For this review, take the finished solid that the model builds, in its own axes (mm). A direction names the side the tool comes from. Coordinates: 2 decimals unless noted, no trailing zeros. Loops run counter-clockwise (first coordinate to the right, second up) from the corner with the lowest first, then second, coordinate; pieces in that order, holes last. Notation, with made-up numbers: M 34,-6.5 L 89,-6.5 A13 cw 89,13.5 Z; hole C 18,79 d10. An arc over 180 degrees is marked long. Write item = value, one per line.
from build123d import *

# Parameters (mm, degrees)
F0_W     = 285
F0_H     = 185
F0_R     = 17.5
F1_DEPTH = 25
F2_SIZE  = 15
F3_T     = -1.5


with BuildPart() as f1:
    # F0 (on Top) → F1 (new body)
    with BuildSketch(Plane.XY):
        with Locations((-142.5, 92.5)):
            Rectangle(F0_W, F0_H)
        with Locations((-142.5, 92.5)):
            Circle(F0_R, mode=Mode.SUBTRACT)
    extrude(amount=F1_DEPTH)

    # F2
    f2_edges = [f1.edges().sort_by_distance(p)[0] for p in [
        (0, 92.5, 25),
        (-142.5, 185, 25),
        (-285, 92.5, 25),
        (-142.5, 0, 25),
    ]]
    chamfer(f2_edges, length=F2_SIZE)

    # F3
    f3_openings = [f1.faces().sort_by_distance(p)[0] for p in [
        (-142.5, 3.397793, 0),
        (-160, 92.5, 12.5),
    ]]
    offset(amount=F3_T, openings=f3_openings)


solid = f1.part
Q1. Draft analysis for pull direction X (two halves, no side actions). For faces 3 (the face through (-144, 185, 5)), 4 (the face through (-277, 91, 18)), 5 (the face through (-144.47, 8.66, 16.54)), 6 (the face through (-8.66, 91.23, 16.54)), state which applies: +X half, -X half, draft (parallel to the pull), parting line (faces both ways), or undercut.
Solved:
face_3 = draft
face_4 = -X half
face_5 = undercut
face_6 = undercut
Q2. Add section D-D (y = 138). Write out the cut boundary in (x, z).
Solved:
outline = M -285,0 L -283.5,0 L -283.5,9.38 L -269.38,23.5 L -15.62,23.5 L -1.5,9.38 L -1.5,0 L 0,0 L 0,10 L -15,25 L -270,25 L -285,10 Z
Q3. For line 1 along Y through (x, z) = (-233.5, 4); line 2 along X through (y, z) = (11.5, 3.25); line 3 along Z through (x, y) = (-238.5, 87), list the stretches that pass through material, from the lowest coordinate up.
Solved:
line_1 = 0 to 1.5, 183.5 to 185
line_2 = -285 to -283.5, -1.5 to 0
line_3 = 23.5 to 25
Q4. Add section C-C (x = -243). Write out the cut boundary in (y, z).
Solved:
outline = M 0,0 L 1.5,0 L 1.5,9.38 L 15.62,23.5 L 169.38,23.5 L 183.5,9.38 L 183.5,0 L 185,0 L 185,10 L 170,25 L 15,25 L 0,10 Z
Q5. Add section B-B (y = 92.5). Write out the cut boundary in (x, z).
Solved:
outline = M -285,0 L -283.5,0 L -283.5,9.38 L -269.38,23.5 L -160,23.5 L -160,25 L -270,25 L -285,10 Z; M -125,23.5 L -15.62,23.5 L -1.5,9.38 L -1.5,0 L 0,0 L 0,10 L -15,25 L -125,25 Z
Q6. Add section A-A (x = -142.5). Write out the cut boundary in (y, z), and give its area (3 significant figures).
Solved:
outline = M 0,0 L 1.5,0 L 1.5,9.38 L 15.62,23.5 L 75,23.5 L 75,25 L 15,25 L 0,10 Z; M 110,23.5 L 169.38,23.5 L 183.5,9.38 L 183.5,0 L 185,0 L 185,10 L 170,25 L 110,25 Z
area = 270 mm²
Q7. For pin 1 Ø4 at (x, y) = (-75, 80) entering from -Z; pin 2 Ø10 at (x, z) = (-190, 20.5) entering from +Y; pin 3 Ø6 at (x, z) = (-141.5, 17) entering from +Y, all flat-tipped, find the tip position at first contact; note any pin that passes through.
Solved:
pin_1 = 23.5
pin_2 = 179.5
pin_3 = 181
Q8. Machinability: for faces 1 (the face through (-144, 111, 25)), 2 (the face through (-283.5, 91, 5)), which of the approach directions +Z, -Z, +X, -X, +Y, -Y give a long, thin tool a straight path to every point of the face, cutting with its end or side? Answer none if there is none.
Solved:
face_1 = +Z, +X, -X, +Y, -Y
face_2 = -Z
